Here's the drawing with two shaded views (mm, measured from the low corner). I have some questions. Coordinates: 2 decimals unless noted, no trailing zeros. Write each loop counter-clockwise with the first axis right and the second up, starting at its lowest first coordinate (ties: lowest second). Pieces come first, ordered by that corner, then holes.
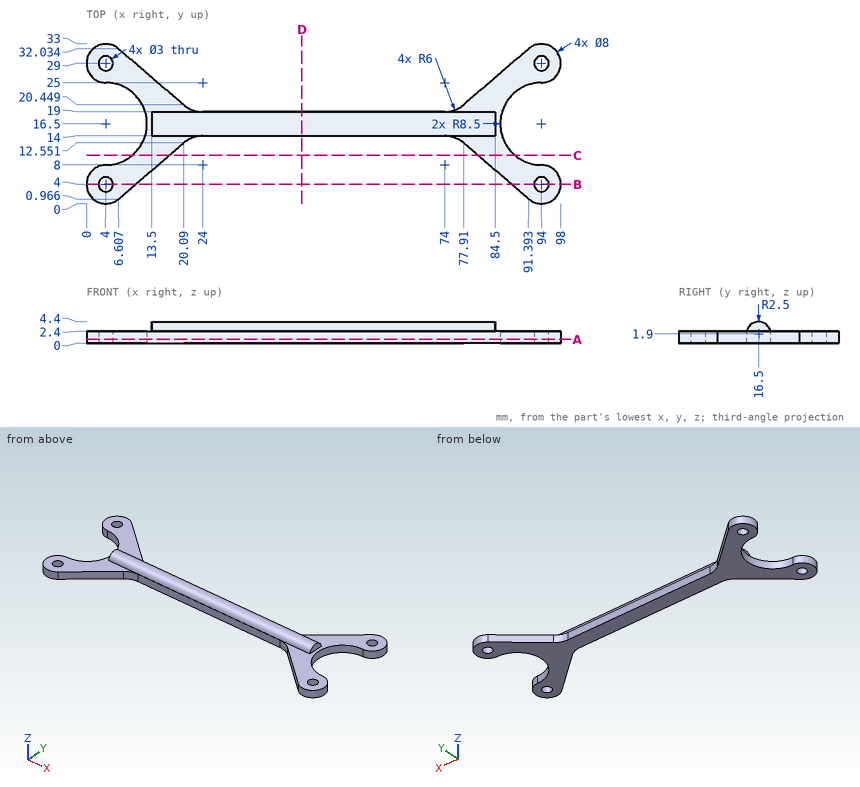
1. I want a section at B-B on y = 4. Please give me the cut outline in (x, z).
Verdict:
outline: (0, 0) - (2.5, 0) - (2.5, 2.4) - (0, 2.4) - close; (5.5, 0) - (10.14, 0) - (10.14, 2.4) - (5.5, 2.4) - close; (87.86, 0) - (92.5, 0) - (92.5, 2.4) - (87.86, 2.4) - close; (95.5, 0) - (98, 0) - (98, 2.4) - (95.5, 2.4) - close
2. Please list where these lines run through material, in increasing order: line 1 along Y through (x, z) = (4, 0.95); line 2 along X through (y, z) = (29, 0.5); line 3 along Y through (x, z) = (27, 1.15).
Verdict:
line 1: y = 0 to 2.5, 5.5 to 8, 25 to 27.5, 30.5 to 33
line 2: x = 0 to 2.5, 5.5 to 10.14, 87.86 to 92.5, 95.5 to 98
line 3: y = 14 to 19
3. I want a section at D-D on x = 44.5. Please give me the cut outline in (y, z).
Verdict:
outline: (14, 0) - (19, 0) - (19, 2.4) - (18.95, 2.4) arc R2.5 ccw to (14.05, 2.4) - (14, 2.4) - close
4. I want a section at A-A on z = 0.75. Please give me the cut outline in (x, y).
Verdict:
outline: (4, 8) arc R4 ccw (long way) to (6.61, 0.97) - (20.09, 12.55) arc R6 cw to (24, 14) - (74, 14) arc R6 cw to (77.91, 12.55) - (91.39, 0.97) arc R4 ccw (long way) to (94, 8) arc R8.5 cw to (94, 25) arc R4 ccw (long way) to (91.39, 32.03) - (77.91, 20.45) arc R6 cw to (74, 19) - (24, 19) arc R6 cw to (20.09, 20.45) - (6.61, 32.03) arc R4 ccw (long way) to (4, 25) arc R8.5 cw to start; hole circle Ø3 at (4, 4); hole circle Ø3 at (4, 29); hole circle Ø3 at (94, 4); hole circle Ø3 at (94, 29)
5. For pin 1 (2 mm diameter, centred on x = 86.5, z = 3.5, fed in from +Y); pin 2 (4 mm diameter, centred on x = 4, y = 29, fed in from +Z); pin 3 (1.6 mm diameter, centred on y = 17, z = 4, fed in from -X); pin 4 (1.5 mm diameter, centred on x = 23, z = 1.5, fed in from +Y), each with a flat end and sliding along its axis, tell me the tip position at first contact or that it passes through.
Verdict:
pin 1: passes through
pin 2: stops at z = 2.4
pin 3: stops at x = 13.5
pin 4: stops at y = 19.26
6. I want a section at C-C on y = 10. Please give me the cut outline in (x, z), plus the area to 3 significant figures.
Verdict:
outline: (9.48, 0) - (17.12, 0) - (17.12, 2.4) - (9.48, 2.4) - close; (80.88, 0) - (88.52, 0) - (88.52, 2.4) - (80.88, 2.4) - close
area: 36.7 mm2
